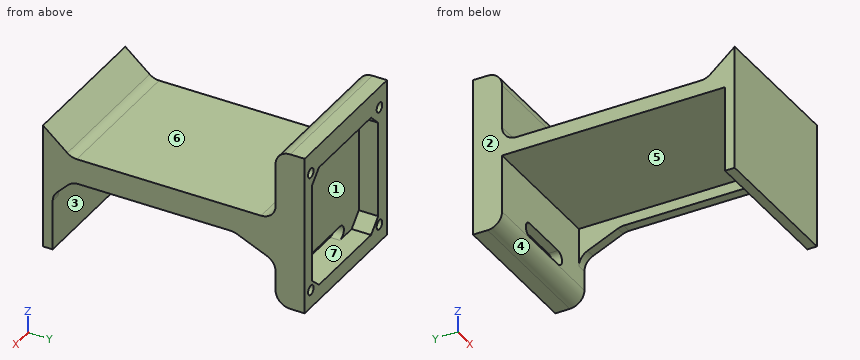
```python
from build123d import *

# Parameters (mm, degrees)
SKETCH_1_W           = 30
SKETCH_1_H           = 50
EXTRUDE_1_DEPTH      = 3
EXTRUDE_2_DEPTH      = 30
EXTRUDE_3_DEPTH      = 15
EXTRUDE_3_DEPTH_BACK = 18
SKETCH_3_W           = 3.207439814
SKETCH_3_H           = 4
SKETCH_3_W_2         = 2.592560186
SKETCH_4_W           = 33
SKETCH_4_H           = 2
EXTRUDE_4_DEPTH      = 30
EXTRUDE_5_DEPTH      = 4
CUT_EXTRUDE_1_DEPTH  = 5
SKETCH_7_R           = 1
SKETCH_7_R_2         = 0.983708166
CUT_EXTRUDE_2_DEPTH  = 5
FILLET_1_R           = 3
FILLET_2_R           = 3
EXTRUDE_6_DEPTH      = 2
FILLET_3_R           = 3
FILLET_4_R           = 3


with BuildPart() as part:
    # 草图1 → 凸台-拉伸1 (new body)
    with BuildSketch(Plane.XY):
        with Locations((-0.718788486, 5)):
            Rectangle(SKETCH_1_W, SKETCH_1_H)
    extrude(amount=EXTRUDE_1_DEPTH)

    # 草图2 → 凸台-拉伸2 (add)
    with BuildSketch(Plane.ZY.offset(15.718788486)):
        Polygon((0, -18.003627417), (-17.838069007, -18.003627417), (-17.838069007, -20), (8.023023193, -20), (3, -14.134137312), align=None)
    extrude(amount=-EXTRUDE_2_DEPTH)

    # 草图3 → 凸台-拉伸3 (add, two sides: drawn at the far end of the back side and taken through both)
    with BuildSketch(Plane.XY.offset(3).offset(-EXTRUDE_3_DEPTH_BACK)):
        with Locations((-14.115068579, 32)):
            Rectangle(SKETCH_3_W, SKETCH_3_H)
        with Locations((12.984931421, 32)):
            Rectangle(SKETCH_3_W_2, SKETCH_3_H)
    extrude(amount=EXTRUDE_3_DEPTH + EXTRUDE_3_DEPTH_BACK)

    # 草图4 → 凸台-拉伸4 (add)
    with BuildSketch(Plane.ZY.offset(15.718788486)):
        with Locations((1.5, 29)):
            Rectangle(SKETCH_4_W, SKETCH_4_H)
    extrude(amount=-EXTRUDE_4_DEPTH)

    # 草图5 → 凸台-拉伸5 (add)
    with BuildSketch(Plane(origin=(0, 30, 0), x_dir=(1, 0, 0), z_dir=(0, 1, 0))):
        Polygon((11.688651328, -18), (-12.511348672, -18), (-12.511348672, -10.700066454), (-9.911348672, -13.250066454), (9.088651328, -13.250066454), (11.688651328, -10.700066454), align=None)
        Polygon((-12.511348672, 15), (-12.511348672, 9.252839713), (-9.911348672, 11.813752042), (9.088651328, 11.813752042), (11.688651328, 9.466986357), (11.688651328, 12.549933546), (11.688651328, 15), align=None)
    extrude(amount=EXTRUDE_5_DEPTH)

    # 草图6 → 切除-拉伸1 (cut)
    with BuildSketch(Plane(origin=(0, 30, 0), x_dir=(1, 0, 0), z_dir=(0, 1, 0))):
        with BuildLine():
            Line((4.654057322, 8.877034891), (-5.604351552, 8.877034891))
            ThreePointArc((-5.604351552, 8.877034891), (-7.072710128, 10.345393466), (-5.604351552, 11.813752042))
            Line((-5.604351552, 11.813752042), (4.654057322, 11.813752042))
            ThreePointArc((4.654057322, 11.813752042), (6.122415898, 10.345393466), (4.654057322, 8.877034891))
        make_face()
    extrude(amount=-CUT_EXTRUDE_1_DEPTH, mode=Mode.SUBTRACT)

    # 草图7 → 切除-拉伸2 (cut)
    with BuildSketch(Plane(origin=(0, 34, 0), x_dir=(1, 0, 0), z_dir=(0, 1, 0))):
        with Locations(Location((-12.963376937, -13.707969551, 0), (0, 0, 270))):
            Circle(SKETCH_7_R)
        with Locations(Location((12.036623063, -13.707969551, 0), (0, 0, 270))):
            Circle(SKETCH_7_R_2)
        with Locations(Location((12.036623063, 11.292030449, 0), (0, 0, 270))):
            Circle(SKETCH_7_R)
        with Locations(Location((-12.963376937, 11.292030449, 0), (0, 0, 270))):
            Circle(SKETCH_7_R)
    extrude(amount=-CUT_EXTRUDE_2_DEPTH, mode=Mode.SUBTRACT)

    # 圆角1
    fillet_1_edges = [part.edges().sort_by_distance(p)[0] for p in [
        (-0.718788486, 28, -15),
        (-0.718788486, 28, 18),
    ]]
    fillet(fillet_1_edges, radius=FILLET_1_R)

    # 圆角2
    fillet_2_edges = [part.edges().sort_by_distance(p)[0] for p in [
        (-0.718788486, 28, 3),
    ]]
    fillet(fillet_2_edges, radius=FILLET_2_R)

    # 草图11 → 凸台-拉伸6 (add)
    with BuildSketch(Plane(origin=(14.281211514, 0, 0), x_dir=(0, 0, -1), z_dir=(1, 0, 0))):
        Polygon((6, 28), (2.205685264, 19.382557308), (2.205685264, -13.954926573), (6.254386108, -18.003627417), (0, -18.003627417), (0, 28), align=None)
    extrude(amount=-EXTRUDE_6_DEPTH)

    # 圆角3
    fillet_3_edges = [part.edges().sort_by_distance(p)[0] for p in [
        (13.281211514, 28, -6),
        (13.281211514, 19.382557308, -2.205685264),
        (13.281211514, -13.954926573, -2.205685264),
        (13.281211514, -18.003627417, -6.254386108),
    ]]
    fillet(fillet_3_edges, radius=FILLET_3_R)

    # 圆角4
    fillet_4_edges = [part.edges().sort_by_distance(p)[0] for p in [
        (-0.718788486, -14.134137312, 3),
    ]]
    fillet(fillet_4_edges, radius=FILLET_4_R)


solid = part.part
```
Here's how the part is built. I have some questions about the finished solid (model axes, mm). Face numbers are marked on the shaded views. A direction names the side the tool comes from. Round coordinates to 2 decimals unless told otherwise and drop trailing zeros. Order: outer loops, then holes, each group sorted by start corner. A loop starts at its lowest first (then second) coordinate and runs counter-clockwise, first axis right, second up. Notation, with made-up numbers: M -29.5,43 L -16.5,43 A26 ccw -16.5,70 Z; hole C 62,62.5 d3. An arc over 180 degrees is marked long. Use CSV: the item, a comma, the result in double quotes.
1) I want a section at A-A (x = 2.75). List the corners of the cut face in (y, z) for me.
Taken from the geometry:
outline,"M -20,-17.84 L -18,-17.84 L -18,0 L 28,0 L 28,-8.88 L 30,-8.88 L 30,13.25 L 34,13.25 L 34,18 L 31,18 A3 ccw 28,15 L 28,6 A3 cw 25,3 L -13.03,3 A3 cw -14.98,3.72 L -20,8.02 Z; M 28,-12 A3 ccw 31,-15 L 34,-15 L 34,-11.81 L 28,-11.81 Z"
2) On a 3-axis mill with a long thin cutter (end or side, diameter ignored), from which of +Z, -Z, +X, -X, +Y, -Y can I reach the whole of each face in a straight line? I mean the marked faces 4, 5, 6 and 7. Say none if no direction works.
Taken from the geometry:
face 4,"-Z, +X, -X"
face 5,"-Z, -X"
face 6,"+Z, +X, -X"
face 7,"+Y"
3) I need wall thicknesses on line 1 along Y through (x, z) = (-1.5, -12); line 2 along X through (y, z) = (30.5, -11); line 3 along Y through (x, z) = (-6.5, -2). Which ranges of each line are inside material? Lowest first, please. Write a range as [from, to].
Taken from the geometry:
line 1,"[-20, -18], [28, 34]"
line 2,"[-15.72, -13.92], [-12.01, -10.74], [9.99, 11.08], [12.99, 14.28]"
line 3,"[-20, -18], [28, 30]"
4) I want a section at B-B (z = 9). List the corners of the cut face in (x, y) for me.
Taken from the geometry:
outline,"M -15.72,28 L 14.28,28 L 14.28,34 L 11.69,34 L 11.69,30 L -12.51,30 L -12.51,34 L -15.72,34 Z"
5) I want a section at D-D (x = -8.25). List the corners of the cut face in (y, z) for me, then the cut area to 3 significant figures.
Taken from the geometry:
outline,"M -20,-17.84 L -18,-17.84 L -18,0 L 28,0 L 28,-12 A3 ccw 31,-15 L 34,-15 L 34,-11.81 L 30,-11.81 L 30,13.25 L 34,13.25 L 34,18 L 31,18 A3 ccw 28,15 L 28,6 A3 cw 25,3 L -13.03,3 A3 cw -14.98,3.72 L -20,8.02 Z"
area,"290 mm^2"
6) I'm going to push flat-ended pins straight in: P1, Ø5, axis at x = 3, z = 5.5, coming from the +Y side; P2, Ø1.2, axis at x = 12.04, z = -11.29, coming from the +Y side; P3, Ø0.6, axis at x = 0.5, y = 28.5, coming from the -Z side. Where does each tip first touch, or does it pass through?
Taken from the geometry:
P1,"y = 30"
P2,"y = 29"
P3,"z = -14.04"
7) I want a section at C-C (y = -2.5). List the corners of the cut face in (x, z) for me.
Taken from the geometry:
outline,"M -15.72,0 L 12.28,0 L 12.28,-2.21 L 14.28,-2.21 L 14.28,3 L -15.72,3 Z"
8) If we mould it in two halves opening along Y, with no side actions, what happens to the marked faces 1, 2 and 3? For each: pulls with the +Y half, pulls with the -Y half, needs draft (parallel to the pull), parting line crosses it, or undercut.
Taken from the geometry:
face 1,"pulls with the +Y half"
face 2,"needs draft"
face 3,"undercut"
